from build123d import *

# Parameters (mm, degrees)
SKETCH_1_W          = 20
SKETCH_1_H          = 12
SKETCH_1_R          = 2.1
SKETCH_1_R_2        = 3.5
EXTRUDE_1_DEPTH     = 2
SKETCH_2_R          = 0.9
SKETCH_2_R_2        = 0.7
CUT_EXTRUDE_1_DEPTH = 24.409399821
CUT_EXTRUDE_START   = 2
SKETCH_2_3_R        = 1.5
CUT_EXTRUDE_2_DEPTH = 1
SKETCH_2_4_R        = 1
CUT_EXTRUDE_3_DEPTH = 1
SKETCH_5_R          = 0.4
CUT_EXTRUDE_4_DEPTH = 24.59745749


with BuildPart() as part:
    # 草图1 → 凸台-拉伸1 (new body)
    with BuildSketch(Plane(origin=(0, 0, 0), x_dir=(1, 0, 0), z_dir=(0, 1, 0))):
        with Locations((10, -6)):
            Rectangle(SKETCH_1_W, SKETCH_1_H)
        with Locations(Location((5, -6, 0), (0, 0, 270))):
            Circle(SKETCH_1_R, mode=Mode.SUBTRACT)
        with Locations(Location((15, -6, 0), (0, 0, 270))):
            Circle(SKETCH_1_R_2, mode=Mode.SUBTRACT)
    extrude(amount=EXTRUDE_1_DEPTH)

    # 草图2 → 切除-拉伸1 (cut, through all)
    with BuildSketch(Plane(origin=(0, 0, 0), x_dir=(1, 0, 0), z_dir=(0, 1, 0))):
        with Locations(Location((2.3, -2.214171161, 0), (0, 0, 270))):
            Circle(SKETCH_2_R)
        with Locations(Location((7.7, -9.785828839, 0), (0, 0, 270))):
            Circle(SKETCH_2_R)
        with Locations(Location((11.5, -1.5, 0), (0, 0, 270))):
            Circle(SKETCH_2_R_2)
        with Locations(Location((18.5, -10.5, 0), (0, 0, 270))):
            Circle(SKETCH_2_R_2)
        with Locations(Location((18.5, -1.5, 0), (0, 0, 270))):
            Circle(SKETCH_2_R_2)
        with Locations(Location((11.5, -10.5, 0), (0, 0, 270))):
            Circle(SKETCH_2_R_2)
    extrude(amount=CUT_EXTRUDE_1_DEPTH, mode=Mode.SUBTRACT)

    # 草图2<3> → 切除-拉伸2 (cut)
    with BuildSketch(Plane(origin=(0, 0, 0), x_dir=(1, 0, 0), z_dir=(0, 1, 0)).offset(CUT_EXTRUDE_START)):
        with Locations(Location((2.3, -2.214171161, 0), (0, 0, 270))):
            Circle(SKETCH_2_3_R)
        with Locations(Location((7.7, -9.785828839, 0), (0, 0, 270))):
            Circle(SKETCH_2_3_R)
    extrude(amount=-CUT_EXTRUDE_2_DEPTH, mode=Mode.SUBTRACT)

    # 草图2<4> → 切除-拉伸3 (cut)
    with BuildSketch(Plane(origin=(0, 0, 0), x_dir=(1, 0, 0), z_dir=(0, 1, 0)).offset(CUT_EXTRUDE_START)):
        with Locations(Location((11.5, -1.5, 0), (0, 0, 270))):
            Circle(SKETCH_2_4_R)
        with Locations(Location((18.5, -10.5, 0), (0, 0, 270))):
            Circle(SKETCH_2_4_R)
        with Locations(Location((18.5, -1.5, 0), (0, 0, 270))):
            Circle(SKETCH_2_4_R)
        with Locations(Location((11.5, -10.5, 0), (0, 0, 270))):
            Circle(SKETCH_2_4_R)
    extrude(amount=-CUT_EXTRUDE_3_DEPTH, mode=Mode.SUBTRACT)

    # 草图5 → 切除-拉伸4 (cut, through all)
    with BuildSketch(Plane(origin=(5, -15.2, 6), x_dir=(0, 0, -1), z_dir=(0, 1, 0))):
        with Locations(Location((0, 3.5, 0), (0, 0, 180))):
            Circle(SKETCH_5_R)
        with Locations(Location((-4.7, -10, 0), (0, 0, 180))):
            Circle(SKETCH_5_R)
        with Locations(Location((4.7, -10, 0), (0, 0, 180))):
            Circle(SKETCH_5_R)
    extrude(amount=CUT_EXTRUDE_4_DEPTH, mode=Mode.SUBTRACT)


solid = part.part
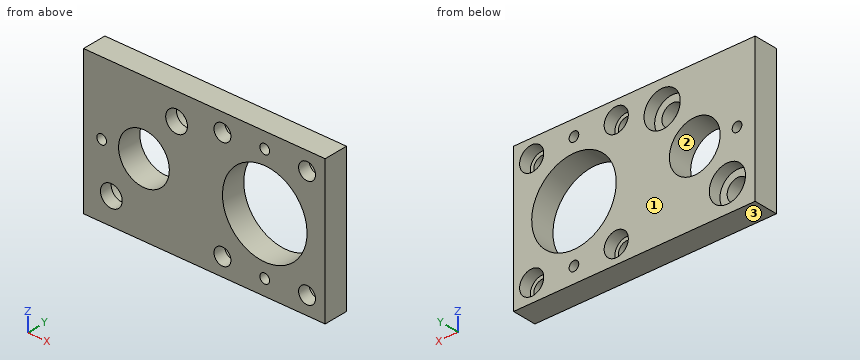
Design review of the part built by this model. Coordinates are the model's own, in mm. Face numbers are marked on the shaded views. Round coordinates to 2 decimals unless told otherwise and drop trailing zeros. Loops run counter-clockwise (first coordinate to the right, second up) from the corner with the lowest first, then second, coordinate; pieces in that order, holes last. Notation, with made-up numbers: (7, 38.5) - (55, 38.5) arc R22 cw to (55, 49.5) - close; hole circle Ø11 at (67.25, -27.5). An arc over 180 degrees is marked (long way). One line per item, written item: value. Start each with the question number.
1) To check wall thickness, follow L1, parallel to Z at x = 19, y = 1.5; L2, parallel to X at y = 1.25, z = 9; L3, parallel to X at y = 0.7, z = 7.25. State the ranges of each line that lie inside material, in increasing order. Write a range as from..to.
2) Draft analysis for pull direction Z (two halves, no side actions). For the marked faces 1, 2 and 3, state which applies: +Z half, -Z half, draft (parallel to the pull), parting line (faces both ways), or undercut.
3) Consider section A-A on x = 7.7. Give the boundary of the cut face in (y, z).
4) Consider section C-C on x = 15. Give the boundary of the cut face in (y, z), then the cut area to 3 significant figures.
5) Consider section B-B on y = 0.75. Give the number of separate pieces and of enclosed holes in the cut face, then the cut area to 3 significant figures.
6) Insertion check: pin 1 Ø1.3 at (x, z) = (18.5, 10.5) entering from -Y; pin 2 Ø1.6 at (x, z) = (18.5, 1.5) entering from -Y. Each pin has a flat end and moves straight along its axis. Give the tip position at first contact, or say it passes through.
7) Consider section D-D on z = 3.5. Give the boundary of the cut face in (x, y).
Reported:
1. L1: z = 0..0.63, 2.37..9.63, 11.37..12
1. L2: x = 0..6.42, 8.98..13.2, 16.8..20
1. L3: x = 0..3.31, 6.69..11.73, 18.27..20
2. face 1: draft
2. face 2: undercut
2. face 3: -Z half
3. outline: (0, 0) - (2, 0) - (2, 8.29) - (1, 8.29) - (1, 8.89) - (0, 8.89) - close; (0, 10.69) - (1, 10.69) - (1, 11.29) - (2, 11.29) - (2, 12) - (0, 12) - close
4. outline: (0, 0) - (2, 0) - (2, 0.9) - (0, 0.9) - close; (0, 1.7) - (2, 1.7) - (2, 2.5) - (0, 2.5) - close; (0, 9.5) - (2, 9.5) - (2, 10.3) - (0, 10.3) - close; (0, 11.1) - (2, 11.1) - (2, 12) - (0, 12) - close
4. area: 6.80 mm^2
5. separate pieces: 1
5. enclosed holes: 11
5. area: 175 mm^2
6. pin 1: passes through
6. pin 2: stops at y = 0
7. outline: (0, 0) - (12.55, 0) - (12.55, 2) - (3.07, 2) - (3.07, 1) - (1.53, 1) - (1.53, 2) - (0, 2) - close; (17.45, 0) - (20, 0) - (20, 2) - (17.45, 2) - close
